The model under review builds one solid part; all positions refer to its coordinate system, in mm. A direction names the side the tool comes from. Round coordinates to 2 decimals unless told otherwise and drop trailing zeros. Write each loop counter-clockwise with the first axis right and the second up, starting at its lowest first coordinate (ties: lowest second). Pieces come first, ordered by that corner, then holes. Notation, with made-up numbers: M 22,73 L 41,73 A38 cw 41,112 Z; hole C 12.5,81.5 d10. An arc over 180 degrees is marked long. One line per item, written item: value. Start each with the question number.
1) Mouldability with a two-part tool opening along Y and no side actions: class faces 4 (the face through (-59.32, -40, 2)), 5 (the face through (37.5, 0, 2)), 6 (the face through (0, -57, 2)) as +Y half, -Y half, draft (parallel to the pull), parting line (faces both ways), or undercut.
2) Wall thickness on probe 1 along Y at (x, z) = (-29, 1.65); probe 2 along X at (y, z) = (-5, 1.75); probe 3 along Y at (x, z) = (-2.5, 1.35): over which ranges is each line inside the solid? List them lowest first.
3) For P1, Ø5, axis at x = -7.5, y = 33, coming from the -Z side; P2, Ø1, axis at y = 68, z = 1.5, coming from the -X side; P3, Ø1, axis at x = 2.5, z = 2, coming from the +Y side; P4, Ø1.6, axis at x = -61.5, z = 2, coming from the +Y side (3 decimals), all flat-tipped, find the tip position at first contact; note any pin that passes through.
4) Take a section at B-B, the plane y = -31. Write out the cut boundary in (x, z).
5) Tool access review of faces 1 (the face through (6, 66.67, 2)), 2 (the face through (-61, -9.875, 2)), 3 (the face through (3.5, -61, 2)): name each direction out of +Z, -Z, +X, -X, +Y, -Y from which nothing blocks a thin tool from reaching the whole face with its end or side.
6) Take a section at A-A, the plane z = 0.9. State how many separate pieces and enclosed holes the cut face has, and give its area (3 significant figures).
from build123d import *

# Parameters (mm, degrees)
SKETCH1_W           = 125
SKETCH1_H           = 140
BOSS_EXTRUDE1_DEPTH = 3.18
SKETCH2_R           = 1.5
SKETCH2_W           = 3.18
SKETCH2_H           = 60.125
SKETCH2_W_2         = 21.82
SKETCH2_H_2         = 64.054089404
SKETCH2_H_3         = 65
CUT_EXTRUDE1_DEPTH  = 4.18
SKETCH12_W          = 35
SKETCH12_H          = 45
CUT_EXTRUDE6_DEPTH  = 4.18
SKETCH13_W          = 15
SKETCH13_H          = 25
CUT_EXTRUDE7_DEPTH  = 4.18
CUT_EXTRUDE11_DEPTH = 10


with BuildPart() as part:
    # Sketch1 → Boss-Extrude1 (new body)
    with BuildSketch(Plane.XY):
        Rectangle(SKETCH1_W, SKETCH1_H)
    extrude(amount=BOSS_EXTRUDE1_DEPTH)

    # Sketch2 → Cut-Extrude1 (cut, through all)
    with BuildSketch(Plane.XY.offset(3.18)):
        with Locations((-60.5, 0)):
            Circle(SKETCH2_R)
        with Locations((85.5, 0)):
            Circle(SKETCH2_R)
        with Locations((-60.91, 39.9375)):
            Rectangle(SKETCH2_W, SKETCH2_H)
        with Locations((-60.91, -39.9375)):
            Rectangle(SKETCH2_W, SKETCH2_H)
        with Locations((73.41, -41.902044702)):
            Rectangle(SKETCH2_W_2, SKETCH2_H_2)
        with Locations((73.41, 42.625)):
            Rectangle(SKETCH2_W_2, SKETCH2_H_3)
        Polygon((1.5, -66.82), (10, -66.82), (10, -70), (-10, -70), (-10, -66.82), (-1.5, -66.82), (-1.5, -62.82), (-3.5, -62.82), (-3.5, -59.82), (-1.5, -59.82), (-1.5, -57), (1.5, -57), (1.5, -59.82), (3.5, -59.82), (3.5, -62.82), (1.5, -62.82), align=None)
    extrude(amount=-CUT_EXTRUDE1_DEPTH, mode=Mode.SUBTRACT)

    # Sketch12 → Cut-Extrude6 (cut, through all)
    with BuildSketch(Plane(origin=(0, 0, 0), x_dir=(-1, 0, 0), z_dir=(0, 0, -1))):
        with Locations((31.82, 0)):
            Rectangle(SKETCH12_W, SKETCH12_H)
    extrude(amount=-CUT_EXTRUDE6_DEPTH, mode=Mode.SUBTRACT)

    # Sketch13 → Cut-Extrude7 (cut, through all)
    with BuildSketch(Plane(origin=(0, 0, 0), x_dir=(-1, 0, 0), z_dir=(0, 0, -1))):
        with Locations((-30, 0)):
            Rectangle(SKETCH13_W, SKETCH13_H)
    extrude(amount=-CUT_EXTRUDE7_DEPTH, mode=Mode.SUBTRACT)

    # Sketch11 → Cut-Extrude11 (cut)
    with BuildSketch(Plane(origin=(0, 0, 0), x_dir=(-1, 0, 0), z_dir=(0, 0, -1))):
        Polygon((-10, 66.67), (-1.5, 66.67), (-1.5, 62.67), (-3.5, 62.67), (-3.5, 59.67), (-1.5, 59.67), (-1.5, 57), (1.5, 57), (1.5, 59.67), (3.5, 59.67), (3.5, 62.67), (1.5, 62.67), (1.5, 66.67), (10, 66.67), (10, 70), (-10, 70), align=None)
    extrude(amount=-CUT_EXTRUDE11_DEPTH, mode=Mode.SUBTRACT)


solid = part.part
Checked values:
1. face 4: draft
1. face 5: undercut
1. face 6: -Y half
2. probe 1: y = -70 to -22.5, 22.5 to 70
2. probe 2: x = -62.5 to -49.32, -14.32 to 22.5, 37.5 to 62.5
2. probe 3: y = -66.82 to -62.82, -59.82 to 59.67, 62.67 to 66.67
3. P1: stops at z = 0
3. P2: stops at x = -59.32
3. P3: stops at y = 66.67
3. P4: stops at y = 9.875
4. outline: M -59.32,0 L 62.5,0 L 62.5,3.18 L -59.32,3.18 Z
5. face 1: +Z, -Z, +Y
5. face 2: +Z, -Z, -X, -Y
5. face 3: +Z, -Z
6. separate pieces: 1
6. enclosed holes: 3
6. area: 14,900 mm2
